Could you check a few things on this model? Use its own coordinates, in mm. A direction names the side the tool comes from. Give positions to 0.01 mm unless a question says otherwise; leave off trailing zeros. Order: outer loops, then holes, each group sorted by start corner. A loop starts at its lowest first (then second) coordinate and runs counter-clockwise, first axis right, second up. Notation, with made-up numbers: (8.5, 46) - (39.5, 46) arc R21 ccw to (39.5, 82) - close; hole circle Ø1 at (-24, -29). An arc over 180 degrees is marked (long way). Put each result on its own line as item: value.
from build123d import *

# Parameters (mm, degrees)
F0_W     = 99.7983887792
F0_H     = 69.3145208061
F1_DEPTH = 50
F2_W     = 48.5056806356
F2_H     = 26.864730753
F3_DEPTH = 100
F7_W     = 31.8869445473
F7_H     = 14.6304946393
F8_DEPTH = 10


with BuildPart() as f1:
    # F0 (on Top) → F1 (new body)
    with BuildSketch(Plane.XY):
        with Locations((5.7157240808, -1.1794362217)):
            Rectangle(F0_W, F0_H)
    extrude(amount=F1_DEPTH)

    # F2 (on face) → F3 (cut)
    with BuildSketch(Plane.XZ.offset(35.8366966248)):
        with Locations((4.7271503136, 25.766398292)):
            Rectangle(F2_W, F2_H)
    extrude(amount=-F3_DEPTH, mode=Mode.SUBTRACT)

    # F7 (on face) → F8 (cut)
    with BuildSketch(Plane.XY.offset(50)):
        with Locations((3.0299229547, -11.6131016985)):
            Rectangle(F7_W, F7_H)
    extrude(amount=-F8_DEPTH, mode=Mode.SUBTRACT)


solid = f1.part
1) Suppose I cut it at C-C, the plane y = -15. List the corners of the cut face in (x, z) for me.
Filled in:
outline: (-44.18, 0) - (55.61, 0) - (55.61, 50) - (18.97, 50) - (18.97, 40) - (-12.91, 40) - (-12.91, 50) - (-44.18, 50) - close; hole (-19.53, 12.33) - (28.98, 12.33) - (28.98, 39.2) - (-19.53, 39.2) - close
2) Suppose I cut it at D-D, the plane z = 47. List the corners of the cut face in (x, y) for me, and give its area (3 significant figures).
Filled in:
outline: (-44.18, -35.84) - (55.61, -35.84) - (55.61, 33.48) - (-44.18, 33.48) - close; hole (-12.91, -18.93) - (18.97, -18.93) - (18.97, -4.3) - (-12.91, -4.3) - close
area: 6,450 mm^2
3) We'd pull the mould along Z, two halves only. Please class faces 1 (the flat face through (5, -1, 0)), 2 (the flat face through (4, -2, 39.199)), 3 (the flat face through (3, -18.928, 45)), 4 (the flat face through (5, -1, 50)): pulls with the +Z half, pulls with the -Z half, needs draft (parallel to the pull), parting line crosses it, or undercut.
Filled in:
face 1: pulls with the -Z half
face 2: undercut
face 3: needs draft
face 4: pulls with the +Z half
4) I'm going to push a flat-ended pin straight in: pin 1 (4.5 mm diameter, centred on x = 7.5, y = -10, fed in from +Z). Where does the tip first touch, or does it pass through?
Filled in:
pin 1: stops at z = 40
5) If I drill on line 1 (X direction, y = -4.5, z = 13); line 2 (Z direction, x = 14.5, y = -0.5); line 3 (Z direction, x = -1, y = -12.5), over which ranges is the centre line in solid material (lowest first)? Write a range as [from, to].
Filled in:
line 1: x = [-44.18, -19.53], [28.98, 55.61]
line 2: z = [0, 12.33], [39.2, 50]
line 3: z = [0, 12.33], [39.2, 40]
6) Suppose I cut it at B-B, the plane z = 29.5. List the corners of the cut face in (x, y) for me, and give its area (3 significant figures).
Filled in:
outline: (-44.18, -35.84) - (-19.53, -35.84) - (-19.53, 33.48) - (-44.18, 33.48) - close; (28.98, -35.84) - (55.61, -35.84) - (55.61, 33.48) - (28.98, 33.48) - close
area: 3,560 mm^2
7) Suppose I cut it at A-A, the plane x = 24. List the corners of the cut face in (y, z) for me, and give its area (3 significant figures).
Filled in:
outline: (-35.84, 0) - (33.48, 0) - (33.48, 12.33) - (-35.84, 12.33) - close; (-35.84, 39.2) - (33.48, 39.2) - (33.48, 50) - (-35.84, 50) - close
area: 1,600 mm^2
8) Which directions (+Z, -Z, +X, -X, +Y, -Y) give clear straight access to the entire face, cutting with the end or side of a thin tool? Please do faces 5 (the flat face through (4, -2, 12.334)), 6 (the flat face through (5, 33.478, 41)), 7 (the flat face through (3, -12, 40)).
Filled in:
face 5: +Y, -Y
face 6: +Z, -Z, +X, -X, +Y
face 7: +Z
